Read the model definition and answer for the solid it produces. Units are mm, in the model's axes. Coordinates: 2 decimals unless noted, no trailing zeros. Write each loop counter-clockwise with the first axis right and the second up, starting at its lowest first coordinate (ties: lowest second). Pieces come first, ordered by that corner, then holes. Notation, with made-up numbers: (49.25, 13) -> (101.25, 13) arc R14 cw to (101.25, 35) -> close; hole circle Ø3 at (69, -4.5). An arc over 180 degrees is marked (long way). One line per item, written item: value. Start each with the question number.
1. Find section B-B, the plane y = 0. Write down the section's boundary in (x, z).
2. Find section A-A, the plane z = 0. Write down the section's boundary in (x, y).
3. For a pull along Z with two mould halves and no side action, classify faces 1 (the flat face through (49, -11, -50)), 2 (the flat face through (0, -11, 23)), 3 (the cylindrical face through (50.7, -4.336, -19.524)) as pulls with the +Z half, pulls with the -Z half, needs draft (parallel to the pull), parting line crosses it, or undercut.
4. Consider line 1 along Z through (x, y) = (46, 0); line 2 along Y through (x, z) = (25.5, -5.5); line 3 along Y through (x, z) = (48, 10). Determine where each line is inside the solid, lowest interval first.
```python
from build123d import *

# Parameters (mm, degrees)
F0_W     = 1000
F0_H     = 100
F1_DEPTH = 100
F2_R     = 20
F3_DEPTH = 100


with BuildPart() as f1:
    # F0 (on Right) → F1 (new body)
    with BuildSketch(Plane.YZ):
        with Locations((-3.763909, 0)):
            Rectangle(F0_W, F0_H)
    extrude(amount=F1_DEPTH)

    # F2 (on face) → F3 (cut)
    with BuildSketch(Plane.YZ.offset(100)):
        Circle(F2_R)
    extrude(amount=-F3_DEPTH, mode=Mode.SUBTRACT)


solid = f1.part
```
Answer block:
1. outline: (0, -50) -> (100, -50) -> (100, -20) -> (0, -20) -> close; (0, 20) -> (100, 20) -> (100, 50) -> (0, 50) -> close
2. outline: (0, -503.76) -> (100, -503.76) -> (100, -20) -> (0, -20) -> close; (0, 20) -> (100, 20) -> (100, 496.24) -> (0, 496.24) -> close
3. face 1: pulls with the -Z half
3. face 2: needs draft
3. face 3: undercut
4. line 1: z = -50 to -20, 20 to 50
4. line 2: y = -503.76 to -19.23, 19.23 to 496.24
4. line 3: y = -503.76 to -17.32, 17.32 to 496.24
